The listing builds one solid part. Answer for the finished solid, in the listing's coordinates (mm). A direction names the side the tool comes from. Coordinates: 2 decimals unless noted, no trailing zeros. Write each loop counter-clockwise with the first axis right and the second up, starting at its lowest first coordinate (ties: lowest second). Pieces come first, ordered by that corner, then holes.
(1) The part is cut by section C-C on z = 1.25. Determine the outline of the cut face in (x, y) (3 decimals).
(2) Which of the six approach directions +Z, -Z, +X, -X, +Y, -Y give full straight-line access (tool end or side, diameter ignored) to faces 4 (the flat face through (23, -35, 5)), 5 (the cylindrical face through (-28.48, -44.27, 2.46)), 6 (the flat face through (-18, -53, 2))?
(3) For a pull along X with two mould halves and no side action, classify faces 1 (the cylindrical face through (37.964, 38.742, 2.535)), 2 (the cylindrical face through (29.564, 27.313, 7.465)), 3 (the flat face through (-37.2, -19.52, 3.82)) as +X half, -X half, draft (parallel to the pull), parting line (faces both ways), or undercut.
(4) Straight lines are drawn through the part: line 1 (Y direction, x = -1, z = 6); line 2 (Z direction, x = 22, y = 36); line 3 (Y direction, x = 34, z = 9.75). For each, find the intervals that lie inside material, in ascending order.
(5) Given P1, Ø2, axis at y = 7, z = 1.5, coming from the -X side; P2, Ø3, axis at x = 31.82, y = -31.82, coming from the +Z side; P3, Ø10, axis at x = -1, y = 29, coming from the +Z side; P4, Ø5, axis at x = -6.5, z = 3.5, coming from the +Y side, each flat-ended and moving along its own axis, determine where each tip first touches the part or whether it passes through.
(6) The part is cut by section D-D on y = 41.5. Determine the outline of the cut face in (x, z).
(7) The part is cut by section A-A on y = 0. Determine the outline of the cut face in (x, z), plus the area to 4 significant figures.
from build123d import *

# Parameters (mm, degrees)
PAD004_DEPTH  = 10
SKETCH001_R   = 40.25
SKETCH001_R_2 = 37
PAD005_DEPTH  = 10
SKETCH_W      = 106
SKETCH_H      = 106
SKETCH_R      = 1.1
SKETCH_R_2    = 37
PAD_DEPTH     = 5
FILLET_1_R    = 50
FILLET_2_R    = 15


with BuildPart() as pad_encoder_hole:
    # Sketch006 → Pad004 (new body)
    with BuildSketch(Plane.XY):
        with BuildLine():
            ThreePointArc((-42.900661, -31.83444), (-44.269937, -28.528716), (-42.900661, -25.222992))
            Line((-42.900661, -25.222992), (-31.955387, -14.277718))
            ThreePointArc((-31.955387, -14.277718), (-24.748737, -24.748737), (-14.277718, -31.955387))
            Line((-14.277718, -31.955387), (-25.222992, -42.900661))
            ThreePointArc((-25.222992, -42.900661), (-28.528716, -44.269937), (-31.83444, -42.900661))
            Line((-31.83444, -42.900661), (-42.900661, -31.83444))
        make_face()
    extrude(amount=PAD004_DEPTH)


with BuildPart() as pad_ring:
    # Sketch001 → Pad005 (new body)
    with BuildSketch(Plane.XY):
        Circle(SKETCH001_R)
        Circle(SKETCH001_R_2, mode=Mode.SUBTRACT)
    extrude(amount=PAD005_DEPTH)


with BuildPart() as fillet_remove_material:
    # Sketch → Pad (new body)
    with BuildSketch(Plane.XY):
        Rectangle(SKETCH_W, SKETCH_H)
        with Locations((-31.819805, 31.819805)):
            Circle(SKETCH_R, mode=Mode.SUBTRACT)
        with Locations((31.819805, 31.819805)):
            Circle(SKETCH_R, mode=Mode.SUBTRACT)
        with Locations((31.819805, -31.819805)):
            Circle(SKETCH_R, mode=Mode.SUBTRACT)
        with Locations((-31.819805, -31.819805)):
            Circle(SKETCH_R, mode=Mode.SUBTRACT)
        Circle(SKETCH_R_2, mode=Mode.SUBTRACT)
    extrude(amount=PAD_DEPTH)

    # Fusion: union Pad (ring)
    add(pad_ring.part)

    # Cut: cut Pad (encoder hole)
    add(pad_encoder_hole.part, mode=Mode.SUBTRACT)

    # Fillet 1
    fillet_1_edges = [fillet_remove_material.edges().sort_by_distance(p)[0] for p in [
        (-53, 53, 2.5),
        (53, 53, 2.5),
        (53, -53, 2.5),
    ]]
    fillet(fillet_1_edges, radius=FILLET_1_R)

    # Fillet 2
    fillet_2_edges = [fillet_remove_material.edges().sort_by_distance(p)[0] for p in [
        (-53, -53, 2.5),
    ]]
    fillet(fillet_2_edges, radius=FILLET_2_R)


solid = fillet_remove_material.part
Model answer:
1. outline: (-53, -38) arc R15 ccw to (-38, -53) - (3, -53) arc R50 ccw to (53, -3) - (53, 3) arc R50 ccw to (3, 53) - (-3, 53) arc R50 ccw to (-53, 3) - close; hole (-42.901, -31.834) - (-31.834, -42.901) arc R4.675 ccw to (-25.223, -42.901) - (-15.786, -33.464) arc R37 ccw (long way) to (-33.464, -15.786) - (-42.901, -25.223) arc R4.675 ccw to start; hole circle Ø2.2 at (-31.82, 31.82); hole circle Ø2.2 at (31.82, -31.82); hole circle Ø2.2 at (31.82, 31.82)
2. face 4: +Z
2. face 5: +Z, -Z
2. face 6: +Z, -Z, +X, -X, -Y
3. face 1: +X half
3. face 2: parting line
3. face 3: undercut
4. line 1: y = -40.24 to -36.99, 36.99 to 40.24
4. line 2: z = 0 to 5
4. line 3: y = -21.54 to -14.59, 14.59 to 21.54
5. P1: stops at x = -52.91
5. P2: stops at z = 5
5. P3: passes through
5. P4: stops at y = 52.99
6. outline: (-34.9, 0) - (34.9, 0) - (34.9, 5) - (-34.9, 5) - close
7. outline: (-53, 0) - (-37, 0) - (-37, 10) - (-40.25, 10) - (-40.25, 5) - (-53, 5) - close; (37, 0) - (53, 0) - (53, 5) - (40.25, 5) - (40.25, 10) - (37, 10) - close
7. area: 192.5 mm2
